Read the model definition and answer for the solid it produces. Units are mm, in the model's axes. Coordinates: 2 decimals unless noted, no trailing zeros. Order: outer loops, then holes, each group sorted by start corner. A loop starts at its lowest first (then second) coordinate and runs counter-clockwise, first axis right, second up.
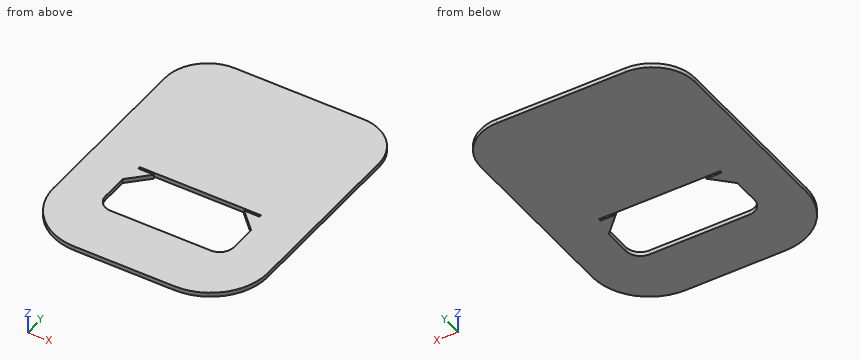
```python
from build123d import *

# Parameters (mm, degrees)
BOSS_EXTRUDE1_DEPTH = 3
SKETCH2_W           = 90
SKETCH2_H           = 44
CUT_EXTRUDE1_DEPTH  = 10
FILLET1_R           = 10
CHAMFER1_SIZE       = 15
SKETCH3_W           = 85
SKETCH3_H           = 1.6
CUT_EXTRUDE2_DEPTH  = 10


with BuildPart() as part:
    # Sketch1 → Boss-Extrude1 (new body)
    with BuildSketch(Plane.XY):
        with BuildLine():
            Line((-45, 96.5), (45, 96.5))
            ThreePointArc((45, 96.5), (66.213203436, 87.713203436), (75, 66.5))
            Line((75, 66.5), (75, -56.5))
            ThreePointArc((75, -56.5), (63.284271247, -84.784271247), (35, -96.5))
            Line((35, -96.5), (0.5, -96.5))
            Line((0.5, -96.5), (-0.5, -96.5))
            Line((-0.5, -96.5), (-35, -96.5))
            ThreePointArc((-35, -96.5), (-63.284271247, -84.784271247), (-75, -56.5))
            Line((-75, -56.5), (-75, 66.5))
            ThreePointArc((-75, 66.5), (-66.213203436, 87.713203436), (-45, 96.5))
        make_face()
    extrude(amount=BOSS_EXTRUDE1_DEPTH)

    # Sketch2 → Cut-Extrude1 (cut)
    with BuildSketch(Plane.XY.offset(3)):
        with Locations((0, -34.5)):
            Rectangle(SKETCH2_W, SKETCH2_H)
    extrude(amount=-CUT_EXTRUDE1_DEPTH, mode=Mode.SUBTRACT)

    # Fillet1
    fillet1_edges = [part.edges().sort_by_distance(p)[0] for p in [
        (45, -56.5, 1.5),
        (-45, -56.5, 1.5),
    ]]
    fillet(fillet1_edges, radius=FILLET1_R)

    # Chamfer1
    chamfer1_edges = [part.edges().sort_by_distance(p)[0] for p in [
        (45, -12.5, 1.5),
        (-45, -12.5, 1.5),
    ]]
    chamfer(chamfer1_edges, length=CHAMFER1_SIZE)

    # Sketch3 → Cut-Extrude2 (cut)
    with BuildSketch(Plane(origin=(0, 0, 0), x_dir=(-1, 0, 0), z_dir=(0, 0, -1))):
        with Locations((0, -13.3)):
            Rectangle(SKETCH3_W, SKETCH3_H)
    extrude(amount=-CUT_EXTRUDE2_DEPTH, mode=Mode.SUBTRACT)


solid = part.part
```
1) A cutting plane is placed at A-A, the plane y = -39. Determine the outline of the cut face in (x, z), and give its area (3 significant figures).
A:
outline: (-75, 0) - (-45, 0) - (-45, 3) - (-75, 3) - close; (45, 0) - (75, 0) - (75, 3) - (45, 3) - close
area: 180 mm2
2) Straight lines are drawn through the part: line 1 (Y direction, x = 5, z = 2.35); line 2 (Y direction, x = 35, z = 0.35); line 3 (Y direction, x = -44, z = 1.3). For each, find the intervals that lie inside material, in ascending order.
A:
line 1: y = -96.5 to -56.5, -12.5 to 96.5
line 2: y = -96.5 to -56.5, -17.5 to -14.1, -12.5 to 96.5
line 3: y = -95.47 to -50.86, -26.5 to 96.5
3) A flat-ended cylindrical pin translates along its axis: pin 1 Ø1 at (x, y) = (-49, -48.5) entering from -Z. Find the tip coordinate at first contact, or state that the pin passes through.
A:
pin 1: stops at z = 0
4) A cutting plane is placed at D-D, the plane x = 55. Determine the outline of the cut face in (y, z), and give its area (3 significant figures).
A:
outline: (-91.14, 0) - (94.78, 0) - (94.78, 3) - (-91.14, 3) - close
area: 558 mm2
5) A cutting plane is placed at B-B, the plane z = 2. Determine the outline of the cut face in (x, y).
A:
outline: (-75, -56.5) arc R40 ccw to (-35, -96.5) - (35, -96.5) arc R40 ccw to (75, -56.5) - (75, 66.5) arc R30 ccw to (45, 96.5) - (-45, 96.5) arc R30 ccw to (-75, 66.5) - close; hole (-45, -46.5) arc R10 ccw to (-35, -56.5) - (35, -56.5) arc R10 ccw to (45, -46.5) - (45, -27.5) - (31.6, -14.1) - (42.5, -14.1) - (42.5, -12.5) - (-42.5, -12.5) - (-42.5, -14.1) - (-31.6, -14.1) - (-45, -27.5) - close
6) A cutting plane is placed at C-C, the plane x = 14.5. Determine the outline of the cut face in (y, z), and give its area (3 significant figures).
A:
outline: (-96.5, 0) - (-56.5, 0) - (-56.5, 3) - (-96.5, 3) - close; (-12.5, 0) - (96.5, 0) - (96.5, 3) - (-12.5, 3) - close
area: 447 mm2
